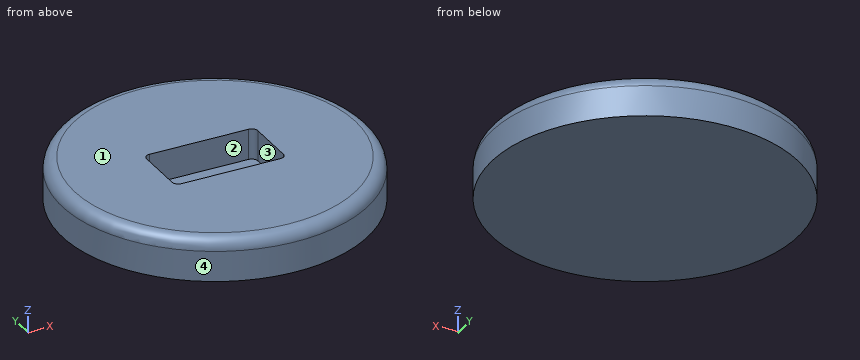
Solid Edge part; units mm, degrees
sketch "Sketch1" plane through (0, 0, 0) normal (0, 0, 1) x (1, 0, 0)
  circle A0 centre (0, 0) radius 25
extrude "Protrusion1" add sketch "Sketch1" along normal blind 7
sketch "Sketch2" plane through (0, 0, 7) normal (0, 0, 1) x (1, 0, 0)
  line L0 (-9.125, -5) -> (9.125, -5)
  line L1 (9.125, -5) -> (9.125, 5)
  line L2 (9.125, 5) -> (-9.125, 5)
  line L3 (-9.125, 5) -> (-9.125, -5)
  dimension "D1" = 9.125
  dimension "D2" = 9.125
extrude "Utskärning_för_pelare" cut sketch "Sketch2" against normal blind 5
fillet "Avrundning_utsida" radius 2 1 edges at (-25, 0, 7)
fillet "Avrundning_insida" radius 1 4 edges at (-9.125, 5, 4.5) (9.125, 5, 4.5) (-9.125, -5, 4.5) (9.125, -5, 4.5)
Geometry: final body of the model. Coordinates: model frame, mm. Face numbers are marked on the shaded views. Coordinates: 2 decimals unless noted, no trailing zeros. Loops run counter-clockwise (first coordinate to the right, second up) from the corner with the lowest first, then second, coordinate; pieces in that order, holes last. Notation, with made-up numbers: (27, 19) - (54, 19) arc R23 ccw to (54, 44) - close; hole circle Ø2 at (-20, 61). An arc over 180 degrees is marked (long way). Put each result on its own line as item: value. Start each with the question number.
Q1. Line query: line 1 (Z direction, x = -1, y = -2.5); line 2 (Y direction, x = -8.5, z = 2.75); line 3 (Z direction, x = 22.5, y = -5.5). Output: solid intervals per line, ascending.
Q2. Cut plane B-B, the plane x = 0. Return loops of the section in (y, z), and give its area (3 significant figures).
Q3. Cut plane C-C, the plane z = 4. Return loops of the section in (x, y) (3 decimals).
Q4. Cut plane A-A, the plane y = 0. Return loops of the section in (x, z) (3 decimals).
Q5. Pull-direction query (Y, two-part tool) for the marked faces 1, 2, 3 and 4; classes: released by +Y, released by -Y, zero draft, split by the parting line, or undercut.
Q6. Pin query (flat end, axial travel): pin 1 Ø3 at (x, y) = (1, -0.5) entering from +Z; pin 2 Ø5 at (x, y) = (1, -19.5) entering from -Z; pin 3 Ø2.5 at (y, z) = (-1.5, 5) entering from -X; pin 4 Ø4 at (x, z) = (-1.5, 5) entering from +Y. Return the tip coordinate at first contact, or that it passes through.
Filled sheet:
1. line 1: 0 to 2
1. line 2: -23.51 to -4.93, 4.93 to 23.51
1. line 3: 0 to 6.99
2. outline: (-25, 0) - (25, 0) - (25, 5) arc R2 ccw to (23, 7) - (5, 7) - (5, 2) - (-5, 2) - (-5, 7) - (-23, 7) arc R2 ccw to (-25, 5) - close
2. area: 298 mm²
3. outline: circle Ø50 at (0, 0); hole (-9.125, -4) arc R1 ccw to (-8.125, -5) - (8.125, -5) arc R1 ccw to (9.125, -4) - (9.125, 4) arc R1 ccw to (8.125, 5) - (-8.125, 5) arc R1 ccw to (-9.125, 4) - close
4. outline: (-25, 0) - (25, 0) - (25, 5) arc R2 ccw to (23, 7) - (9.125, 7) - (9.125, 2) - (-9.125, 2) - (-9.125, 7) - (-23, 7) arc R2 ccw to (-25, 5) - close
5. face 1: zero draft
5. face 2: undercut
5. face 3: undercut
5. face 4: split by the parting line
6. pin 1: z = 2
6. pin 2: z = 0
6. pin 3: x = -25
6. pin 4: y = 25
